Build history of the part. All positions in model axes, mm. Face numbers are marked on the shaded views. A direction names the side the tool comes from. Give positions to 0.01 mm unless a question says otherwise; leave off trailing zeros. Order: outer loops, then holes, each group sorted by start corner. A loop starts at its lowest first (then second) coordinate and runs counter-clockwise, first axis right, second up. Notation, with made-up numbers: (-12, -8) -> (11, -8) arc R24 cw to (11, 14) -> close; hole circle Ø10 at (-23, 9.5). An arc over 180 degrees is marked (long way). Use a Markdown table: item, result. Add a question column.
```python
from build123d import *

# Parameters (mm, degrees)
F1_DEPTH = 3
F2_W     = 33
F2_H     = 3
F2_W_2   = 3
F3_DEPTH = 30
F4_W     = 33
F4_H     = 7
F4_H_2   = 3
F5_DEPTH = 3
F6_W     = 30.5
F6_H     = 30.5
F7_DEPTH = 2


# Not quite as in the source:
# - a feature names something its author has since deleted; it is built from what else it names


with BuildPart() as f1:
    # F0 (on Top) → F1 (new body)
    with BuildSketch(Plane.XY):
        Polygon((17.5, 10.8150299639), (7, 17.5), (-7, 17.5), (-17.5, 10.8150299639), (-17.5, -17.5), (17.5, -17.5), align=None)
    extrude(amount=F1_DEPTH)

    # F2 (on face) → F3 (join)
    with BuildSketch(Plane.XY.offset(3)):
        with Locations((0, -16)):
            Rectangle(F2_W, F2_H)
        with Locations((-15, -9)):
            Rectangle(F2_W_2, F2_H)
        with Locations((15, -9)):
            Rectangle(F2_W_2, F2_H)
    extrude(amount=F3_DEPTH)

    # F4 (on face) → F5 (join)
    with BuildSketch(Plane.XY.offset(33)):
        with Locations((0, -11)):
            Rectangle(F4_W, F4_H)
        with Locations((0, -16)):
            Rectangle(F4_W, F4_H_2)
    extrude(amount=F5_DEPTH)

    # F6 (on face) → F7 (cut)
    with BuildSketch(Plane.XZ.offset(17.5)):
        with Locations((0, 18.25)):
            Rectangle(F6_W, F6_H)
    extrude(amount=-F7_DEPTH, mode=Mode.SUBTRACT)


solid = f1.part
```
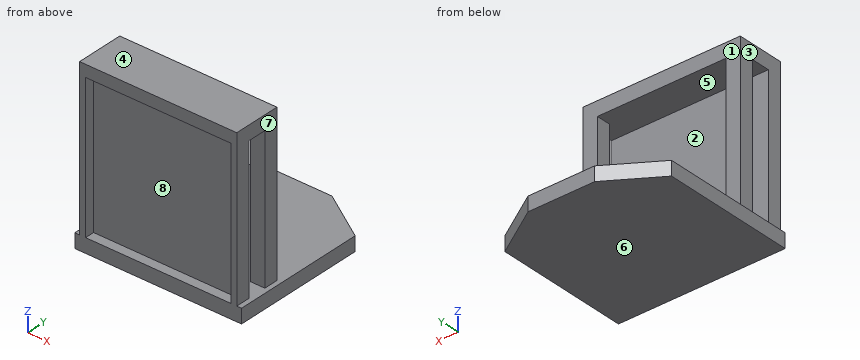
(1) Band-saw the part on B-B on y = -10. Give the cut face in (x, z).
(2) Band-saw the part on D-D on y = 9.5. Give the cut face in (x, z), plus the area to 3 significant figures.
(3) Band-saw the part on C-C on x = -6. Give the cut face in (y, z).
(4) Mould opens along Z. For the marked faces 6, 7 and 8 say: released by +Z, released by -Z, zero draft, split by the parting line, or undercut.
(5) Wall check: probe 1 along Z at (x, y) = (-10.5, -14); probe 2 along Y at (x, z) = (16, 16.5); probe 3 along Y at (x, z) = (14, 28). Give the ranges that are in metal, low to high.
(6) Tool access for the marked faces 1, 2, 3, 4 and 5: list every direction of +Z, -Z, +X, -X, +Y, -Y with a clear straight run to the whole face (end or side of a thin tool).
(7) Pin check, flat tips, straight feed: pin 1 Ø1.5 at (x, z) = (15, 22.5) entering from -Y; pin 2 Ø1.5 at (x, y) = (-8.5, 13.5) entering from +Z; pin 3 Ø0.6 at (y, z) = (-16.5, 12.5) entering from +X; pin 4 Ø2 at (y, z) = (-16, 20) entering from -X. Stop position of each tip, or through.
(8) Band-saw the part on A-A on z = 10.5. Give the cut face in (x, y).
Response:
| question | item | result |
|---|---|---|
| 1 | outline | (-17.5, 0) -> (17.5, 0) -> (17.5, 3) -> (16.5, 3) -> (16.5, 36) -> (-16.5, 36) -> (-16.5, 3) -> (-17.5, 3) -> close; hole (-13.5, 3) -> (13.5, 3) -> (13.5, 33) -> (-13.5, 33) -> close |
| 2 | outline | (-17.5, 0) -> (17.5, 0) -> (17.5, 3) -> (-17.5, 3) -> close |
| 2 | area | 105 mm² |
| 3 | outline | (-17.5, 0) -> (17.5, 0) -> (17.5, 3) -> (-14.5, 3) -> (-14.5, 33) -> (-7.5, 33) -> (-7.5, 36) -> (-17.5, 36) -> (-17.5, 33.5) -> (-15.5, 33.5) -> (-15.5, 3) -> (-17.5, 3) -> close |
| 4 | face 6 | released by -Z |
| 4 | face 7 | zero draft |
| 4 | face 8 | undercut |
| 5 | probe 1 | z = 0 to 3, 33 to 36 |
| 5 | probe 2 | y = -17.5 to -14.5, -10.5 to -7.5 |
| 5 | probe 3 | y = -15.5 to -14.5, -10.5 to -7.5 |
| 6 | face 1 | +Z, +X, -X, +Y |
| 6 | face 2 | +X, -X |
| 6 | face 3 | +Z, -X, +Y, -Y |
| 6 | face 4 | +Z, +X, -X, +Y, -Y |
| 6 | face 5 | none |
| 7 | pin 1 | stops at y = -17.5 |
| 7 | pin 2 | stops at z = 3 |
| 7 | pin 3 | stops at x = 16.5 |
| 7 | pin 4 | stops at x = -16.5 |
| 8 | outline | (-16.5, -17.5) -> (-15.25, -17.5) -> (-15.25, -15.5) -> (15.25, -15.5) -> (15.25, -17.5) -> (16.5, -17.5) -> (16.5, -14.5) -> (-16.5, -14.5) -> close; (-16.5, -10.5) -> (-13.5, -10.5) -> (-13.5, -7.5) -> (-16.5, -7.5) -> close; (13.5, -10.5) -> (16.5, -10.5) -> (16.5, -7.5) -> (13.5, -7.5) -> close |
